Geometry check sheet. Reference: the model listing, model coordinates, mm. A direction names the side the tool comes from. Give positions to 0.01 mm unless a question says otherwise; leave off trailing zeros. Write each loop counter-clockwise with the first axis right and the second up, starting at its lowest first coordinate (ties: lowest second). Pieces come first, ordered by that corner, then holes. Notation, with made-up numbers: (9, -33.5) - (52, -33.5) arc R7 cw to (52, -26.5) - close; hole circle Ø6 at (82, -20.5). An arc over 180 degrees is marked (long way). One line per question, with ' | ' between items. Start each with the question number.
Q1. Section check D-D on z = 45.5. Record the boundary of the cut face in (x, y).
Q2. Release check for a two-part mould opening along X. For faces 1 (the face through (8, 0, 19)), 2 (the face through (-15, 9, 24)), 3 (the face through (-1.658, 57.532, 24.157)), 4 (the face through (2.476, 74.219, 24.843)) record: +X half, -X half, draft (parallel to the pull), parting line (faces both ways), or undercut.
Q3. Section check B-B on y = 65. Record the boundary of the cut face in (x, z).
Q4. Thickness scan on L1, parallel to X at y = -38.5, z = 22.5; L2, parallel to Y at x = 3, z = 31; L3, parallel to Y at x = -8, z = 13. Record the ranges inside material, lowest first. Write a range as [from, to].
Q5. Section check A-A on x = 15. Record the boundary of the cut face in (y, z), and give its area (3 significant figures).
Q6. Section check C-C on z = 5.5. Count the separate pieces of the cut face and the enclosed holes in it, and give its area (3 significant figures).
Q7. Set-up check for faces 5 (the face through (0, 8, 19)), 6 (the face through (27.205, 16.304, 24.157)): record each of +Z, -Z, +X, -X, +Y, -Y from which the full face is reachable in a straight line by a thin tool's end or side.
Q8. Gauge pin test, flat ends, axial feed: P1, Ø2, axis at x = 0, y = 8, coming from the -Z side; P2, Ø2.5, axis at x = 8.5, y = 0, coming from the -Z side. Record the tip position at first contact, or that the pin passes through.
```python
from build123d import *

# Parameters (mm, degrees)
SZKIC1_R                    = 7.65
SZKIC1_R_2                  = 5.3
SZKIC1_R_3                  = 5
DODANIE_WYCI_GNI_CIE1_DEPTH = 49
ZAOKR_GLENIE1_R             = 16
SZKIC2_R                    = 11
WYTNIJ_WYCI_GNI_CIE1_DEPTH  = 4
SZKIC3_R                    = 1.21
WYTNIJ_WYCI_GNI_CIE2_DEPTH  = 15


with BuildPart() as part:
    # Szkic1 → Dodanie-wyciągnięcie1 (new body)
    with BuildSketch(Plane.XY):
        Polygon((-15, -57), (-15, 77), (4.572094065, 77), (54.539400892, -57), align=None)
        with Locations((0, 65)):
            Circle(SZKIC1_R, mode=Mode.SUBTRACT)
        with Locations((0, -45)):
            Circle(SZKIC1_R, mode=Mode.SUBTRACT)
        Circle(SZKIC1_R_2, mode=Mode.SUBTRACT)
        with Locations((15, 29)):
            Circle(SZKIC1_R_3, mode=Mode.SUBTRACT)
        with Locations((39.457289313, -36.58842123)):
            Circle(SZKIC1_R_3, mode=Mode.SUBTRACT)
    extrude(amount=DODANIE_WYCI_GNI_CIE1_DEPTH)

    # Zaokrąglenie1
    zaokr_glenie1_edges = [part.edges().sort_by_distance(p)[0] for p in [
        (4.572094065, 77, 24.5),
        (54.539400892, -57, 24.5),
    ]]
    fillet(zaokr_glenie1_edges, radius=ZAOKR_GLENIE1_R)

    # Szkic2 → Wytnij-wyciągnięcie1 (cut)
    with BuildSketch(Plane(origin=(0, 0, 0), x_dir=(-1, 0, 0), z_dir=(0, 0, -1))):
        Circle(SZKIC2_R)
    extrude(amount=-WYTNIJ_WYCI_GNI_CIE1_DEPTH, mode=Mode.SUBTRACT)

    # Szkic3 → Wytnij-wyciągnięcie2 (cut)
    with BuildSketch(Plane(origin=(0, 0, 4), x_dir=(-1, 0, 0), z_dir=(0, 0, -1))):
        with Locations((0, 8)):
            Circle(SZKIC3_R)
        with Locations((8, 0)):
            Circle(SZKIC3_R)
        with Locations((0, -8)):
            Circle(SZKIC3_R)
        with Locations((-8, 0)):
            Circle(SZKIC3_R)
    extrude(amount=-WYTNIJ_WYCI_GNI_CIE2_DEPTH, mode=Mode.SUBTRACT)


solid = part.part
```
Working result:
1) outline: (-15, -57) - (31.5, -57) arc R16 ccw to (46.49, -35.41) - (8.45, 66.59) arc R16 ccw to (-6.54, 77) - (-15, 77) - close; hole circle Ø15.3 at (0, -45); hole circle Ø15.3 at (0, 65); hole circle Ø10.6 at (0, 0); hole circle Ø10 at (15, 29); hole circle Ø10 at (39.46, -36.59)
2) face 1: undercut | face 2: -X half | face 3: undercut | face 4: +X half
3) outline: (-15, 0) - (-7.65, 0) - (-7.65, 49) - (-15, 49) - close; (7.65, 0) - (9.05, 0) - (9.05, 49) - (7.65, 49) - close
4) L1: x = [-15, -4.03], [4.03, 34.84], [44.08, 47.3] | L2: y = [-57, -52.04], [-37.96, -4.37], [4.37, 57.96], [72.04, 73.85] | L3: y = [-57, -1.21], [1.21, 77]
5) outline: (-57, 0) - (24, 0) - (24, 49) - (-57, 49) - close; (34, 0) - (49.03, 0) - (49.03, 49) - (34, 49) - close | area: 4,710 mm2
6) separate pieces: 1 | enclosed holes: 9 | area: 5,190 mm2
7) face 5: -Z | face 6: +Z, -Z, +X, +Y
8) P1: stops at z = 19 | P2: stops at z = 4
